from build123d import *

# Parameters (mm, degrees)
BOSS_EXTRUDE2_DEPTH = 50
SKETCH19_R          = 4.25
CUT_EXTRUDE4_DEPTH  = 59.449844405
SKETCH20_R          = 11.2
CUT_EXTRUDE5_DEPTH  = 7.2
CUT_EXTRUDE6_START  = -7.2
SKETCH21_R          = 11.2
CUT_EXTRUDE6_DEPTH  = 7.2
SKETCH29_W          = 67.039204955
SKETCH29_H          = 49.809734905
SKETCH29_R          = 3.175
SKETCH29_W_2        = 30
SKETCH29_H_2        = 44.809734905
BOSS_EXTRUDE4_DEPTH = 2


with BuildPart() as part:
    # Sketch11 → Boss-Extrude2 (new body)
    with BuildSketch(Plane(origin=(0, 0, 0), x_dir=(-1, 0, 0), z_dir=(0, 0.08715574274765156, -0.9961946980917461))):
        with BuildLine():
            Line((-17.5, 0), (-17.5, 17.5))
            Line((-17.5, 17.5), (17.5, 17.5))
            Line((17.5, 17.5), (17.5, 0))
            ThreePointArc((17.5, 0), (0, -17.5), (-17.5, 0))
        make_face()
    extrude(amount=BOSS_EXTRUDE2_DEPTH)

    # Sketch19 → Cut-Extrude4 (cut, through all)
    with BuildSketch(Plane(origin=(0, 0, 0), x_dir=(1, 0, 0), z_dir=(0, -0.08715574274765156, 0.9961946980917461))):
        with Locations(Location((0, 0, 0), (0, 0, 270))):
            Circle(SKETCH19_R)
    extrude(amount=-CUT_EXTRUDE4_DEPTH, mode=Mode.SUBTRACT)

    # Sketch20 → Cut-Extrude5 (cut)
    with BuildSketch(Plane(origin=(0, 0, 0), x_dir=(1, 0, 0), z_dir=(0, -0.08715574274765156, 0.9961946980917461))):
        with Locations(Location((0, 0, 0), (0, 0, 270))):
            Circle(SKETCH20_R)
    extrude(amount=-CUT_EXTRUDE5_DEPTH, mode=Mode.SUBTRACT)

    # Sketch21 → Cut-Extrude6 (cut)
    with BuildSketch(Plane(origin=(0, 4.357787137, -49.809734905), x_dir=(-1, 0, 0), z_dir=(0, 0.08715574274765156, -0.9961946980917461)).offset(CUT_EXTRUDE6_START)):
        with Locations(Location((0, 0, 0), (0, 0, 270))):
            Circle(SKETCH21_R)
    extrude(amount=CUT_EXTRUDE6_DEPTH, mode=Mode.SUBTRACT)

    # Sketch23 → Loft3 section 0
    with BuildSketch(Plane(origin=(0, 17.433407217, 1.525225498), x_dir=(1, 0, 0), z_dir=(0, 0.9961946980917462, 0.08715574274765159))):
        with BuildLine():
            Line((17.5, 0), (17.5, 50))
            Line((17.5, 50), (-17.5, 50))
            Line((-17.5, 50), (-17.5, 0))
            Line((-17.5, 0), (17.5, 0))
        make_face()
    # Sketch24 → Loft3 section 1
    with BuildSketch(Plane(origin=(0, 41.791194354, 0), x_dir=(1, 0, 0), z_dir=(0, 1, 0))):
        with BuildLine():
            Line((17.5, -1.525225498), (17.5, 48.284509407))
            Line((17.5, 48.284509407), (-17.5, 48.284509407))
            Line((-17.5, 48.284509407), (-17.5, -1.525225498))
            Line((-17.5, -1.525225498), (17.5, -1.525225498))
        make_face()
    loft()

    # Sketch26 → Cut-Loft7 section 0
    with BuildSketch(Plane(origin=(0, 41.791194354, 0), x_dir=(1, 0, 0), z_dir=(0, 1, 0))):
        with BuildLine():
            Line((-15, 0.974774502), (15, 0.974774502))
            Line((15, 0.974774502), (15, 45.784509407))
            Line((15, 45.784509407), (-15, 45.784509407))
            Line((-15, 45.784509407), (-15, 0.974774502))
        make_face()
    # Sketch27 → Cut-Loft7 section 1
    with BuildSketch(Plane(origin=(0, 21.791194354, 0), x_dir=(1, 0, 0), z_dir=(0, 1, 0))):
        with BuildLine():
            Line((15, 0.974774502), (15, 45.784509407))
            Line((15, 45.784509407), (-15, 45.784509407))
            Line((-15, 45.784509407), (-15, 0.974774502))
            Line((-15, 0.974774502), (15, 0.974774502))
        make_face()
    loft(mode=Mode.SUBTRACT)

    # Cut-Loft8: read off the stored shape, not the designer's step
    # Cut-Loft8: loft between two sections, ruled curve by curve
    cut_loft8_from = [
        Edge.make_bspline([(2.4, 2.52751654, -28.889646245), (2.4, 2.544947688, -29.088885184), (2.37568, 2.564665803, -29.314264273), (2.23232, 2.607504594, -29.803913891), (2.112, 2.630708939, -30.069140767), (1.728, 2.675332679, -30.579192453), (1.461591696, 2.696640901, -30.822746545), (0.963321799, 2.719802012, -31.087479253), (0.781633136, 2.726029473, -31.158659456), (0.399905325, 2.734478939, -31.25523729), (0.2, 2.736690322, -31.28051352), (-0.2, 2.736690322, -31.28051352), (-0.399905325, 2.734478939, -31.25523729), (-0.781633136, 2.726029473, -31.158659456), (-0.963321799, 2.719802012, -31.087479253), (-1.461591696, 2.696640901, -30.822746545), (-1.728, 2.675332679, -30.579192453), (-2.112, 2.630708939, -30.069140767), (-2.23232, 2.607504594, -29.803913891), (-2.37568, 2.564665803, -29.314264273), (-2.4, 2.544947688, -29.088885184), (-2.4, 2.52751654, -28.889646245)], [0, 0, 0, 0, 0.125, 0.125, 0.25, 0.25, 0.375, 0.375, 0.4375, 0.4375, 0.5, 0.5, 0.5625, 0.5625, 0.625, 0.625, 0.75, 0.75, 0.875, 0.875, 1, 1, 1, 1], 3),
        Edge.make_bspline([(-2.4, 2.52751654, -28.889646245), (-2.4, 2.411308883, -27.561386647), (-2.4, 2.295101226, -26.23312705), (-2.4, 2.062685912, -23.576607855), (-2.4, 1.946478255, -22.248348257), (-2.4, 1.830270598, -20.92008866)], [0, 0, 0, 0, 0.5, 0.5, 1, 1, 1, 1], 3),
        Edge.make_bspline([(2.4, 1.830270598, -20.92008866), (2.4, 1.946478255, -22.248348257), (2.4, 2.062685912, -23.576607855), (2.4, 2.295101226, -26.23312705), (2.4, 2.411308883, -27.561386647), (2.4, 2.52751654, -28.889646245)], [0, 0, 0, 0, 0.5, 0.5, 1, 1, 1, 1], 3),
        Edge.make_bspline([(-2.4, 1.830270598, -20.92008866), (-2.4, 1.812839449, -20.72084972), (-2.37568, 1.793121334, -20.495470632), (-2.23232, 1.750282543, -20.005821014), (-2.112, 1.727078198, -19.740594137), (-1.728, 1.682454458, -19.230542452), (-1.461591696, 1.661146236, -18.98698836), (-0.963321799, 1.637985125, -18.722255651), (-0.781633136, 1.631757664, -18.651075448), (-0.399905325, 1.623308199, -18.554497614), (-0.2, 1.621096815, -18.529221385), (0.2, 1.621096815, -18.529221385), (0.399905325, 1.623308199, -18.554497614), (0.781633136, 1.631757664, -18.651075448), (0.963321799, 1.637985125, -18.722255651), (1.461591696, 1.661146236, -18.98698836), (1.728, 1.682454458, -19.230542452), (2.112, 1.727078198, -19.740594137), (2.23232, 1.750282543, -20.005821014), (2.37568, 1.793121334, -20.495470632), (2.4, 1.812839449, -20.72084972), (2.4, 1.830270598, -20.92008866)], [0, 0, 0, 0, 0.125, 0.125, 0.25, 0.25, 0.375, 0.375, 0.4375, 0.4375, 0.5, 0.5, 0.5625, 0.5625, 0.625, 0.625, 0.75, 0.75, 0.875, 0.875, 1, 1, 1, 1], 3),
    ]
    cut_loft8_to = [
        Edge.make_bspline([(15, 21.791194354, -45.784509407), (13.75, 21.791194354, -45.784509407), (12.5, 21.791194354, -45.784509407), (10, 21.791194354, -45.784509407), (8.75, 21.791194354, -45.784509407), (6.25, 21.791194354, -45.784509407), (5, 21.791194354, -45.784509407), (3.125, 21.791194354, -45.784509407), (2.5, 21.791194354, -45.784509407), (1.25, 21.791194354, -45.784509407), (0.625, 21.791194354, -45.784509407), (-0.625, 21.791194354, -45.784509407), (-1.25, 21.791194354, -45.784509407), (-2.5, 21.791194354, -45.784509407), (-3.125, 21.791194354, -45.784509407), (-5, 21.791194354, -45.784509407), (-6.25, 21.791194354, -45.784509407), (-8.75, 21.791194354, -45.784509407), (-10, 21.791194354, -45.784509407), (-12.5, 21.791194354, -45.784509407), (-13.75, 21.791194354, -45.784509407), (-15, 21.791194354, -45.784509407)], [0, 0, 0, 0, 0.125, 0.125, 0.25, 0.25, 0.375, 0.375, 0.4375, 0.4375, 0.5, 0.5, 0.5625, 0.5625, 0.625, 0.625, 0.75, 0.75, 0.875, 0.875, 1, 1, 1, 1], 3),
        Edge.make_bspline([(-15, 21.791194354, -45.784509407), (-15, 21.791194354, -38.316220256), (-15, 21.791194354, -30.847931105), (-15, 21.791194354, -15.911352803), (-15, 21.791194354, -8.443063653), (-15, 21.791194354, -0.974774502)], [0, 0, 0, 0, 0.5, 0.5, 1, 1, 1, 1], 3),
        Edge.make_bspline([(15, 21.791194354, -0.974774502), (15, 21.791194354, -8.443063653), (15, 21.791194354, -15.911352803), (15, 21.791194354, -30.847931105), (15, 21.791194354, -38.316220256), (15, 21.791194354, -45.784509407)], [0, 0, 0, 0, 0.5, 0.5, 1, 1, 1, 1], 3),
        Edge.make_bspline([(-15, 21.791194354, -0.974774502), (-13.75, 21.791194354, -0.974774502), (-12.5, 21.791194354, -0.974774502), (-10, 21.791194354, -0.974774502), (-8.75, 21.791194354, -0.974774502), (-6.25, 21.791194354, -0.974774502), (-5, 21.791194354, -0.974774502), (-3.125, 21.791194354, -0.974774502), (-2.5, 21.791194354, -0.974774502), (-1.25, 21.791194354, -0.974774502), (-0.625, 21.791194354, -0.974774502), (0.625, 21.791194354, -0.974774502), (1.25, 21.791194354, -0.974774502), (2.5, 21.791194354, -0.974774502), (3.125, 21.791194354, -0.974774502), (5, 21.791194354, -0.974774502), (6.25, 21.791194354, -0.974774502), (8.75, 21.791194354, -0.974774502), (10, 21.791194354, -0.974774502), (12.5, 21.791194354, -0.974774502), (13.75, 21.791194354, -0.974774502), (15, 21.791194354, -0.974774502)], [0, 0, 0, 0, 0.125, 0.125, 0.25, 0.25, 0.375, 0.375, 0.4375, 0.4375, 0.5, 0.5, 0.5625, 0.5625, 0.625, 0.625, 0.75, 0.75, 0.875, 0.875, 1, 1, 1, 1], 3),
    ]
    cut_loft8 = Solid(Shell([*[Face.make_surface_from_curves(cut_loft8_from[k], cut_loft8_to[k]) for k in range(4)], Face(Wire(cut_loft8_from)), Face(Wire(cut_loft8_to))]))
    add(cut_loft8, mode=Mode.SUBTRACT)

    # Sketch29 → Boss-Extrude4 (add)
    with BuildSketch(Plane(origin=(0, 41.791194354, 0), x_dir=(1, 0, 0), z_dir=(0, 1, 0))):
        with Locations((0.397406033, 23.379641955)):
            Rectangle(SKETCH29_W, SKETCH29_H)
        with Locations(Location((-28.284271247, 23.474774502, 0), (0, 0, 270))):
            Circle(SKETCH29_R, mode=Mode.SUBTRACT)
        with Locations(Location((28.284271247, 23.474774502, 0), (0, 0, 90))):
            Circle(SKETCH29_R, mode=Mode.SUBTRACT)
        with Locations((0, 23.379641955)):
            Rectangle(SKETCH29_W_2, SKETCH29_H_2, mode=Mode.SUBTRACT)
    extrude(amount=BOSS_EXTRUDE4_DEPTH)


solid = part.part
Geometry: final body of the model. Coordinates: model frame, mm. A direction names the side the tool comes from. Coordinates: 2 decimals unless noted, no trailing zeros. Order: outer loops, then holes, each group sorted by start corner. A loop starts at its lowest first (then second) coordinate and runs counter-clockwise, first axis right, second up.
(1) Access query for faces 1 (the face through (24, 41.791, -24)), 2 (the face through (28.145, 42.777, -20.303)), 3 (the face through (0, 33, -0.975)), 4 (the face through (-17.5, 23, -24)). Directions: +Z, -Z, +X, -X, +Y, -Y. A direction counts if a zero-diameter tool reaches every point of the face in a straight line with its end or side. Return the directions, or none.
(2) Section query B-B (x = -2). State how many separate pieces and enclosed holes the cut face has, plus the area to 3 significant figures.
(3) First-contact query: pin 1 (10 mm diameter, centred on x = -28.28, z = -23.47, fed in from -Y); pin 2 (8 mm diameter, centred on x = 6, z = -15, fed in from -Y); pin 3 (6 mm diameter, centred on x = -13, y = -8, fed in from +Z); pin 4 (2 mm diameter, centred on x = 20, y = 33.5, fed in from +Z). Flat tips, straight axial feed; report the tip coordinate or a pass-through.
(4) Section query A-A (y = 23). Return the cut outline in (x, z).
(5) Draft query along X for faces 5 (the face through (-15, 33, -23)), 6 (the face through (17.5, 23, -23)), 7 (the face through (0, 30, 1.525)). Return one class per face: pulls with the +X half, pulls with the -X half, needs draft (parallel to the pull), parting line crosses it, or undercut.
(6) Material intervals for probe 1 along X at (y, z) = (37.5, -31.5); probe 2 along Z at (x, y) = (-8, 29.5); probe 3 along Y at (x, z) = (-24.5, -16.5), sorted ascending.
(7) Section query C-C (x = 18.5). Return the cut outline in (y, z).
Solution:
1. face 1: +Z, -Z, +X, -Y
1. face 2: +Y, -Y
1. face 3: +Y
1. face 4: +Z, -Z, -X, -Y
2. separate pieces: 3
2. enclosed holes: 0
2. area: 876 mm2
3. pin 1: stops at y = 41.79
3. pin 2: stops at y = -16.24
3. pin 3: stops at z = -0.44
3. pin 4: passes through
4. outline: (-17.5, -48.28) - (17.5, -48.28) - (17.5, 1.53) - (-17.5, 1.53) - close; hole (-15, -45.78) - (15, -45.78) - (15, -0.97) - (-15, -0.97) - close
5. face 5: undercut
5. face 6: pulls with the +X half
5. face 7: needs draft
6. probe 1: x = -17.5 to -15, 15 to 17.5
6. probe 2: z = -48.28 to -45.78, -0.97 to 1.53
6. probe 3: y = 41.79 to 43.79
7. outline: (41.79, -48.28) - (43.79, -48.28) - (43.79, 1.53) - (41.79, 1.53) - close
